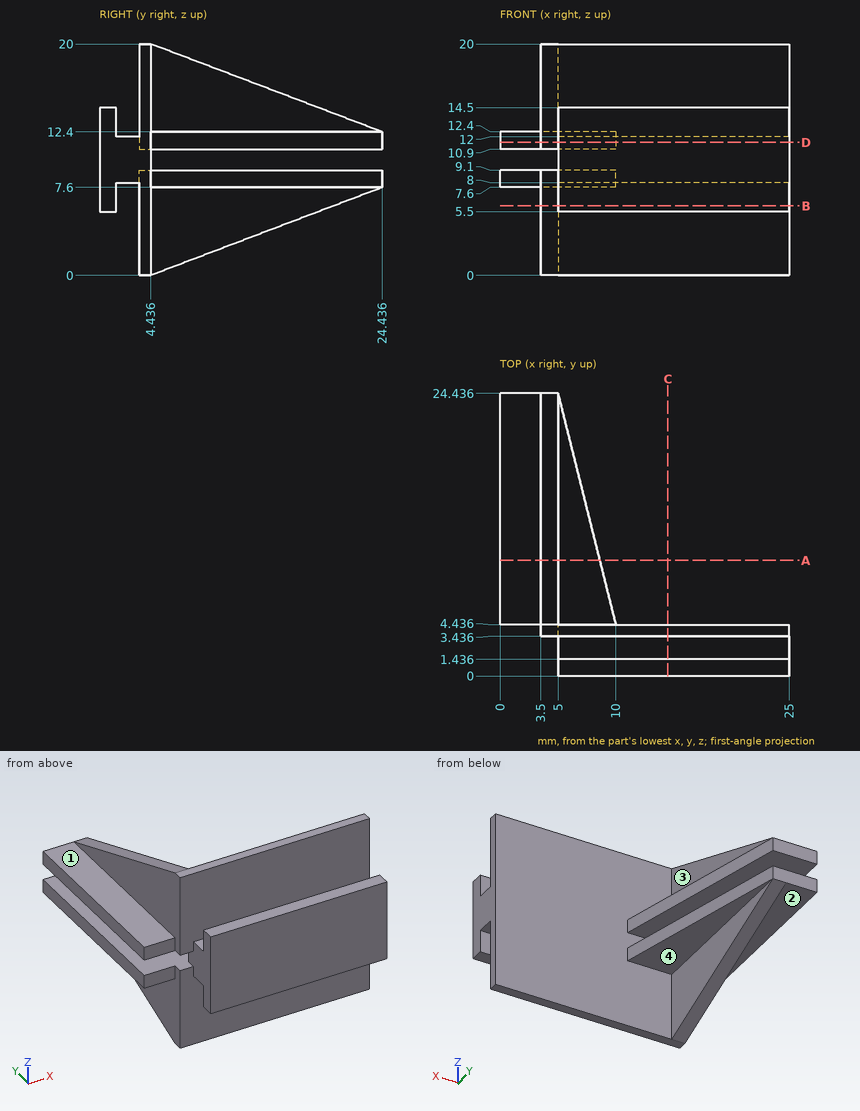
Verification items for this drawing (mm, ordinates from the low corner). A direction names the side the tool comes from. Round coordinates to 2 decimals unless told otherwise and drop trailing zeros. Order: outer loops, then holes, each group sorted by start corner. A loop starts at its lowest first (then second) coordinate and runs counter-clockwise, first axis right, second up. Notation, with made-up numbers: (55.25, 87.5) -> (75.25, 87.5) arc R12 cw to (75.25, 94.5) -> close; hole circle Ø11 at (14.5, 12). An arc over 180 degrees is marked (long way). Use one line per item in the form item = value.
1. Cross-section at B-B, the plane z = 6. Enter the section's corners in (x, y).
Working result:
outline = (3.5, 3.44) -> (25, 3.44) -> (25, 4.44) -> (5, 4.44) -> (5, 20.23) -> (3.5, 20.23) -> close; (5, 0) -> (25, 0) -> (25, 1.44) -> (5, 1.44) -> close
2. Cross-section at C-C, the plane x = 14.5. Enter the section's corners in (y, z), plus the area to 3 significant figures.
Working result:
outline = (0, 5.5) -> (1.44, 5.5) -> (1.44, 8) -> (3.44, 8) -> (3.44, 0) -> (4.44, 0) -> (4.44, 20) -> (3.44, 20) -> (3.44, 12) -> (1.44, 12) -> (1.44, 14.5) -> (0, 14.5) -> close
area = 40.9 mm^2
3. Cross-section at A-A, the plane y = 10. Enter the section's corners in (x, z), plus the area to 3 significant figures.
Working result:
outline = (0, 7.6) -> (3.5, 7.6) -> (3.5, 2.11) -> (5, 2.11) -> (5, 7.6) -> (8.61, 7.6) -> (8.61, 9.1) -> (0, 9.1) -> close; (0, 10.9) -> (8.61, 10.9) -> (8.61, 12.4) -> (5, 12.4) -> (5, 17.89) -> (3.5, 17.89) -> (3.5, 12.4) -> (0, 12.4) -> close
area = 42.3 mm^2
4. Go/stop test with flat-tipped pins: pin 1 (1.2 mm diameter, centred on x = 18, z = 6.5, fed in from +Y); pin 2 (1.6 mm diameter, centred on x = 14, y = 0.5, fed in from -Z); pin 3 (1.6 mm diameter, centred on x = 2.5, z = 8.5, fed in from -Y). Record where each tip stops, or that it passes through.
Working result:
pin_1 = 4.44
pin_2 = 5.5
pin_3 = 4.44
5. Cross-section at D-D, the plane z = 11.5. Enter the section's corners in (x, y), plus the area to 3 significant figures.
Working result:
outline = (0, 4.44) -> (3.5, 4.44) -> (3.5, 3.44) -> (5, 3.44) -> (5, 0) -> (25, 0) -> (25, 4.44) -> (10, 4.44) -> (5, 24.44) -> (0, 24.44) -> close
area = 240 mm^2
6. Set-up check for the marked faces 1, 2, 3 and 4: record each of +Z, -Z, +X, -X, +Y, -Y from which the full face is reachable in a straight line by a thin tool's end or side.
Working result:
face_1 = +Z, -X, +Y, -Y
face_2 = -Z, -X, +Y, -Y
face_3 = +Z, +X, +Y
face_4 = -Z, +X, +Y
7. Scan lines: line 1 along Y through (x, z) = (13.5, 6.5); line 2 along Y through (x, z) = (23, 15.5); line 3 along Z through (x, y) = (7.75, 5.25). Record each from-to range of solid material in increasing order. Write a range as from..to.
Working result:
line_1 = 0..1.44, 3.44..4.44
line_2 = 3.44..4.44
line_3 = 7.6..9.1, 10.9..12.4
